Here's how the part is built. I have some questions about the finished solid (model axes, mm). A direction names the side the tool comes from. Give positions to 0.01 mm unless a question says otherwise; leave off trailing zeros. Write each loop counter-clockwise with the first axis right and the second up, starting at its lowest first coordinate (ties: lowest second). Pieces come first, ordered by that corner, then holes. Notation, with made-up numbers: (-18.75, -25.5) - (-3.75, -25.5) arc R15 ccw to (-3.75, -18.5) - close; hole circle Ø4 at (-26.5, 68). An arc over 180 degrees is marked (long way). Use a Markdown table: item, result.
```python
from build123d import *

# Parameters (mm, degrees)
SKETCH1_W                   = 56.388
SKETCH1_H                   = 6.35
BOSS_EXTRUDE1_DEPTH         = 3.175
F_17_0_173_DIAMETER_HOLE1_D = 4.3942
SKETCH4_W                   = 47.244
SKETCH4_H                   = 2.286
CUT_EXTRUDE1_DEPTH          = 30.074125283


with BuildPart() as part:
    # Sketch1 → Boss-Extrude1 (new, symmetric)
    with BuildSketch(Plane(origin=(0, 0, 0), x_dir=(1, 0, 0), z_dir=(0, 1, 0))):
        Rectangle(SKETCH1_W, SKETCH1_H)
    extrude(amount=BOSS_EXTRUDE1_DEPTH, both=True)

    # #17 (0.173) Diameter Hole1 (through all)
    with Locations(Plane(origin=(0, 3.175, 0), x_dir=(1, 0, 0), z_dir=(0, 1, 0))):
        with Locations((-23.622, 0)):
            Hole(F_17_0_173_DIAMETER_HOLE1_D / 2)

    # Sketch4 → Cut-Extrude1 (cut, through all)
    with BuildSketch(Plane(origin=(0, 3.175, 0), x_dir=(1, 0, 0), z_dir=(0, 1, 0))):
        with Locations((4.572, 2.032)):
            Rectangle(SKETCH4_W, SKETCH4_H)
    cut_extrude1 = extrude(amount=-CUT_EXTRUDE1_DEPTH, mode=Mode.SUBTRACT)

    # Mirror1: Cut-Extrude1 across plane
    add(cut_extrude1.mirror(Plane.XY), mode=Mode.SUBTRACT)


solid = part.part
```
Item 1: For faces 4 (the flat face through (4, 0, -0.889)), 5 (the flat face through (28.194, 0, 0)), which set-ups out of +Z, -Z, +X, -X, +Y, -Y let a thin tool reach every point of the face, with its end or its side?
Values:
| item | result |
|---|---|
| face 4 | -Z, +X, +Y, -Y |
| face 5 | +Z, -Z, +X, +Y, -Y |
Item 2: If we section it at B-B, the plane y = -1.5: Write out the boundary of the cut face in (x, z) (3 decimals).
Values:
| item | result |
|---|---|
| outline | (-28.194, -3.175) - (-19.05, -3.175) - (-19.05, -0.889) - (28.194, -0.889) - (28.194, 0.889) - (-19.05, 0.889) - (-19.05, 3.175) - (-28.194, 3.175) - close; hole circle Ø4.394 at (-23.622, 0) |
Item 3: I need wall thicknesses on line 1 along Z through (x, y) = (-13, -1.25); line 2 along X through (y, z) = (1.75, 0.75); line 3 along X through (y, z) = (0.5, -1). Which ranges of each line are inside material? Lowest first, please. Write a range as [from, to].
Values:
| item | result |
|---|---|
| line 1 | z = [-0.89, 0.89] |
| line 2 | x = [-28.19, -25.69], [-21.56, 28.19] |
| line 3 | x = [-28.19, -25.58], [-21.67, -19.05] |
Item 4: Thinking about a two-plate mould opening in X: for faces 1 (the flat face through (4, 0, 0.889)), 2 (the flat face through (-19.05, 0, 2)), 3 (the cylindrical face through (-25.652, -0.044, 0.842)), which applies, +X half, -X half, draft (parallel to the pull), parting line (faces both ways), or undercut?
Values:
| item | result |
|---|---|
| face 1 | draft |
| face 2 | +X half |
| face 3 | undercut |
Item 5: If we section it at A-A, the plane z = 0: Write out the boundary of the cut face in (x, y) (3 decimals).
Values:
| item | result |
|---|---|
| outline | (-28.194, -3.175) - (-25.819, -3.175) - (-25.819, 3.175) - (-28.194, 3.175) - close; (-21.425, -3.175) - (28.194, -3.175) - (28.194, 3.175) - (-21.425, 3.175) - close |
Item 6: If we section it at C-C, the plane x = -14.5: Write out the boundary of the cut face in (y, z) (3 decimals), plus the area to 3 significant figures.
Values:
| item | result |
|---|---|
| outline | (-3.175, -0.889) - (3.175, -0.889) - (3.175, 0.889) - (-3.175, 0.889) - close |
| area | 11.3 mm2 |
Item 7: Will these pins go through, and if not, where does the flat tip stop? pin 1 Ø3 at (x, y) = (11.5, 1.5) entering from +Z; pin 2 Ø1.5 at (y, z) = (0.5, 2) entering from +X; pin 3 Ø2.5 at (y, z) = (-1, -2) entering from +X; pin 4 Ø1.9 at (x, y) = (6.5, -1.5) entering from -Z.
Values:
| item | result |
|---|---|
| pin 1 | stops at z = 0.89 |
| pin 2 | stops at x = -19.05 |
| pin 3 | stops at x = 28.19 |
| pin 4 | stops at z = -0.89 |
